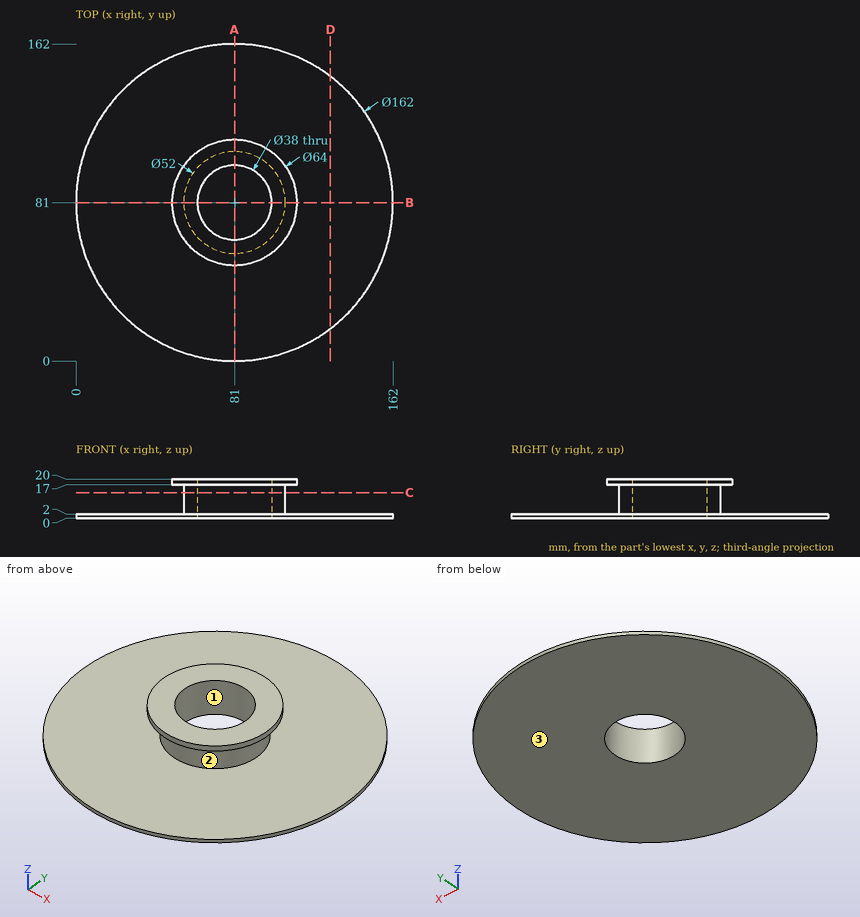
Part print with two shaded views. Sizes in mm from the minimum x, y, z corner. Round coordinates to 2 decimals unless told otherwise and drop trailing zeros. Loops run counter-clockwise (first coordinate to the right, second up) from the corner with the lowest first, then second, coordinate; pieces in that order, holes last. Notation, with made-up numbers: M 55,78.25 L 71,78.25 A29 cw 71,105.25 Z; hole C -5,84.5 d5. An arc over 180 degrees is marked long. Return JSON: item names as keys, results as strings. Group by question number.
(1) Wall check: probe 1 along Y at (x, z) = (81, 6.5); probe 2 along Z at (x, y) = (53.5, 150.5); probe 3 along X at (y, z) = (67, 4.75). Give the ranges that are in metal, low to high. Write a range as [from, to].
(2) Mould opens along X. For the marked faces 1, 2 and 3 say: +X half, -X half, draft (parallel to the pull), parting line (faces both ways), or undercut.
(3) Saw through at D-D, the plane x = 130. List the corners of the cut face in (y, z).
(4) Saw through at C-C, the plane z = 13. List the corners of the cut face in (x, y), and give its area (3 significant figures).
(5) Saw through at A-A, the plane x = 81. List the corners of the cut face in (y, z).
(6) Drop flat-ended pins along their axis: P1, Ø3, axis at y = 91.5, z = 18, coming from the -X side; P2, Ø5, axis at y = 87, z = 12.5, coming from the -X side. Give the stop position or say it passes through.
Answer list:
{
 "1": {"probe 1": "[55, 62], [100, 107]", "probe 2": "[0, 2]", "probe 3": "[59.09, 68.15], [93.85, 102.91]"},
 "2": {"face 1": "undercut", "face 2": "parting line", "face 3": "draft"},
 "3": {"outline": "M 16.5,0 L 145.5,0 L 145.5,2 L 16.5,2 Z"},
 "4": {"outline": "C 81,81 d52; hole C 81,81 d38", "area": "990 mm2"},
 "5": {"outline": "M 0,0 L 62,0 L 62,20 L 49,20 L 49,17 L 55,17 L 55,2 L 0,2 Z; M 100,0 L 162,0 L 162,2 L 107,2 L 107,17 L 113,17 L 113,20 L 100,20 Z"},
 "6": {"P1": "x = 50.29", "P2": "x = 55.24"}
}
